Source: CAD feature listing. Evaluate the final solid. Frame: model axes, mm. Face numbers are marked on the shaded views. A direction names the side the tool comes from. Give positions to 0.01 mm unless a question says otherwise; leave off trailing zeros. Order: outer loops, then holes, each group sorted by start corner. A loop starts at its lowest first (then second) coordinate and runs counter-clockwise, first axis right, second up. Notation, with made-up numbers: M -37.5,86.25 L 18.5,86.25 A15 cw 18.5,94.25 Z; hole C -4,-28 d4. An arc over 180 degrees is marked long. One line per question, with ' | ' between items. Start each with the question number.
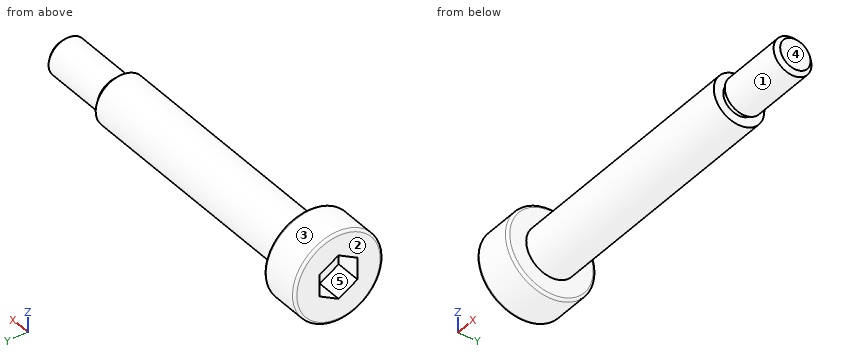
from build123d import *

# Parameters (mm, degrees)
FILLET_1_R          = 0.2
CHAMFER_1_SIZE      = 0.3
SKETCH_3_W          = 0.5
SKETCH_3_H          = 0.25
CUT_EXTRUDE_1_DEPTH = 2


with BuildPart() as part:
    # 草图1 → 旋转1 (revolve)
    with BuildSketch(Plane.XY, mode=Mode.PRIVATE) as revolve_1_sk:
        Polygon((-14.6, 0), (-14.6, 3.5), (-11.4, 3.5), (-11.4, 2), (8.6, 2), (8.6, 1.5), (14.6, 1.5), (14.6, 0), align=None)
    revolve(revolve_1_sk.sketch.rotate(Axis((-14.6, 0, 0), (1, 0, 0)), 90), axis=Axis((-14.6, 0, 0), (1, 0, 0)))

    # 圆角1
    fillet_1_edges = [part.edges().sort_by_distance(p)[0] for p in [
        (-11.4, 0, -3.5),
        (-14.6, 0, -3.5),
    ]]
    fillet(fillet_1_edges, radius=FILLET_1_R)

    # 倒角1
    chamfer_1_edges = [part.edges().sort_by_distance(p)[0] for p in [
        (14.6, 0, -1.5),
    ]]
    chamfer(chamfer_1_edges, length=CHAMFER_1_SIZE)

    # 草图3 → 切除-旋转1 (revolve, cut)
    with BuildSketch(Plane.XY, mode=Mode.PRIVATE) as cut_revolve_1_sk:
        with Locations((8.85, 1.375)):
            Rectangle(SKETCH_3_W, SKETCH_3_H)
    revolve(cut_revolve_1_sk.sketch.rotate(Axis((8.6, 0, 0), (1, 0, 0)), 90), axis=Axis((8.6, 0, 0), (1, 0, 0)), mode=Mode.SUBTRACT)

    # 草图4 → 切除-拉伸1 (cut)
    with BuildSketch(Plane.ZY.offset(14.6)):
        Polygon((1.732050808, 0), (0.866025404, 1.5), (-0.866025404, 1.5), (-1.732050808, 0), (-0.866025404, -1.5), (0.866025404, -1.5), align=None)
    extrude(amount=-CUT_EXTRUDE_1_DEPTH, mode=Mode.SUBTRACT)


solid = part.part
Item 1: Mould query, pull axis Z, two halves, no side actions, for the marked faces 3, 4 and 5. Classes: pulls with the +Z half, pulls with the -Z half, needs draft (parallel to the pull), parting line crosses it, or undercut.
Item 2: Cut plane A-A on z = 0. Return the cut outline in (x, y).
Item 3: Pin query (flat end, axial travel): pin 1 Ø4 at (x, z) = (9, 0) entering from +Y; pin 2 Ø2 at (x, z) = (-9.5, -2.5) entering from +Y; pin 3 Ø0.9 at (x, z) = (-13.5, -0.5) entering from -Y; pin 4 Ø2 at (x, z) = (-3, 1.5) entering from -Y. Return the tip coordinate at first contact, or that it passes through.
Item 4: Line query: line 1 (X direction, y = -2, z = 0.75); line 2 (X direction, y = -1.25, z = 0.5); line 3 (X direction, y = -1.25, z = -1.25). Output: solid intervals per line, ascending.
Item 5: Cut plane B-B on x = -2.5. Return the cut outline in (y, z), and give its area (3 significant figures).
Item 6: Reachability of the marked faces 1 and 2 from +Z, -Z, +X, -X, +Y, -Y: full face, straight path, thin tool, end or side. Return the list, or none.
Results are:
1) face 3: parting line crosses it | face 4: needs draft | face 5: undercut
2) outline: M -14.6,-3.3 A0.2 ccw -14.4,-3.5 L -11.6,-3.5 A0.2 ccw -11.4,-3.3 L -11.4,-2 L 8.6,-2 L 8.6,-1.25 L 9.1,-1.25 L 9.1,-1.5 L 14.3,-1.5 L 14.6,-1.2 L 14.6,1.2 L 14.3,1.5 L 9.1,1.5 L 9.1,1.25 L 8.6,1.25 L 8.6,2 L -11.4,2 L -11.4,3.3 A0.2 ccw -11.6,3.5 L -14.4,3.5 A0.2 ccw -14.6,3.3 L -14.6,1.5 L -12.6,1.5 L -12.6,-1.5 L -14.6,-1.5 Z
3) pin 1: stops at y = 2 | pin 2: stops at y = 1.32 | pin 3: stops at y = -3.5 | pin 4: stops at y = -1.94
4) line 1: x = -14.6 to -11.4 | line 2: x = -12.6 to 8.6, 9.1 to 14.45 | line 3: x = -14.6 to 8.6
5) outline: C 0,0 d4 | area: 12.6 mm2
6) face 1: +X | face 2: +Z, -Z, -X, +Y, -Y
